Here's how the part is built. I have some questions about the finished solid (model axes, mm). Face numbers are marked on the shaded views. A direction names the side the tool comes from. Coordinates: 2 decimals unless noted, no trailing zeros. Write each loop counter-clockwise with the first axis right and the second up, starting at its lowest first coordinate (ties: lowest second). Pieces come first, ordered by that corner, then holes. Notation, with made-up numbers: (79, -29) - (123, -29) arc R22 ccw to (123, -8) - close; hole circle Ø6 at (89.25, 32.25). An arc over 180 degrees is marked (long way). Answer in a Markdown table with one row per item. Add a question column.
Item 1: Which directions (+Z, -Z, +X, -X, +Y, -Y) give clear straight access to the entire face, cutting with the end or side of a thin tool? Please do the marked faces 1 and 2.
Item 2: If I drill on probe 1 along Y at (x, z) = (2.5, 5.25); probe 2 along Y at (x, z) = (2.5, 0.5); probe 3 along X at (y, z) = (14, -0.25), over which ranges is the centre line in solid material (lowest first)? Write a range as from..to.
Item 3: Imagine slicing it at A-A (y = 2). Please give me the cut outline in (x, z), plus the area to 3 significant figures.
Item 4: We'd pull the mould along Y, two halves only. Please class the marked faces 3, 4 and 5: +Y half, -Y half, draft (parallel to the pull), parting line (faces both ways), or undercut.
Item 5: I'm going to push flat-ended pins straight in: pin 1 (2 mm diameter, centred on x = -2.5, z = 4.5, fed in from +Y); pin 2 (0.8 mm diameter, centred on x = 2, z = -3.5, fed in from -Y); pin 3 (2 mm diameter, centred on x = 3, z = 4, fed in from +Y). Where does each tip first touch, or does it pass through?
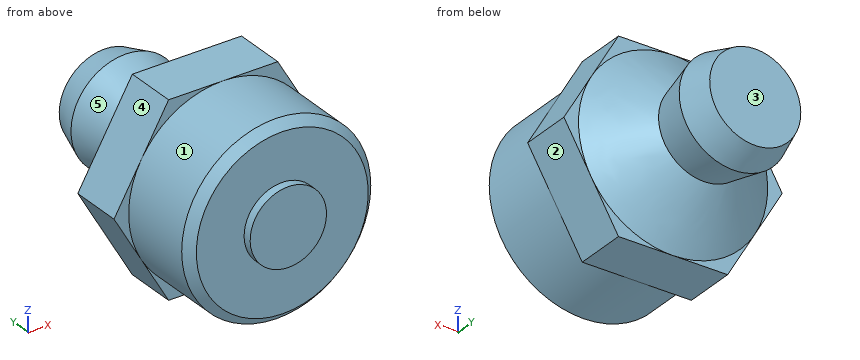
from build123d import *

# Parameters (mm, degrees)
SKETCH1_R           = 5.5
BOSS_EXTRUDE1_DEPTH = 4.89
CHAMFER1_SIZE       = 0.5
SKETCH2_R           = 2.22
BOSS_EXTRUDE2_DEPTH = 0.5
BOSS_EXTRUDE3_DEPTH = 3
SKETCH4_R           = 2.65
BOSS_EXTRUDE4_DEPTH = 2.57
SKETCH8_R           = 3.195
SKETCH5_R           = 2.65


with BuildPart() as part:
    # Sketch1 → Boss-Extrude1 (new body)
    with BuildSketch(Plane(origin=(0, 0, 0), x_dir=(1, 0, 0), z_dir=(0, 1, 0))):
        with Locations(Location((0, 0, 0), (0, 0, 270))):
            Circle(SKETCH1_R)
    extrude(amount=BOSS_EXTRUDE1_DEPTH)

    # Chamfer1
    chamfer1_edges = [part.edges().sort_by_distance(p)[0] for p in [
        (0, 0, -5.5),
    ]]
    chamfer(chamfer1_edges, length=CHAMFER1_SIZE)

    # Sketch2 → Boss-Extrude2 (add)
    with BuildSketch(Plane(origin=(0, 0, 0), x_dir=(-1, 0, 0), z_dir=(0, -1, 0))):
        with Locations(Location((0, 0, 0), (0, 0, 90))):
            Circle(SKETCH2_R)
    extrude(amount=BOSS_EXTRUDE2_DEPTH)

    # Sketch3 → Boss-Extrude3 (add)
    with BuildSketch(Plane(origin=(0, 4.89, 0), x_dir=(1, 0, 0), z_dir=(0, 1, 0))):
        Polygon((-6.350852961, 0), (-3.175426481, -5.5), (3.175426481, -5.5), (6.350852961, 0), (3.175426481, 5.5), (-3.175426481, 5.5), align=None)
    extrude(amount=BOSS_EXTRUDE3_DEPTH)

    # Sketch4 → Boss-Extrude4 (add)
    with BuildSketch(Plane(origin=(0, 7.89, 0), x_dir=(1, 0, 0), z_dir=(0, 1, 0))):
        with Locations(Location((0, 0, 0), (0, 0, 270))):
            Circle(SKETCH4_R)
    extrude(amount=BOSS_EXTRUDE4_DEPTH)

    # Loft1: read off the stored shape, not the designer's step
    # Loft1: loft between two sections, ruled curve by curve
    loft1_from = [
        Edge.make_bspline([(2.920740302, 7.89, 4.660394413), (12.241529129, 7.89, -1.181086191), (6.400048524, 7.89, -10.501875018), (-2.920740302, 7.89, -4.660394413), (-12.241529129, 7.89, 1.181086191), (-6.400048524, 7.89, 10.501875018), (2.920740302, 7.89, 4.660394413)], [0, 0, 0, 0, 0.5, 0.5, 0.5, 1, 1, 1, 1], 3, [1, 0.333333333, 0.333333333, 1, 0.333333333, 0.333333333, 1]),
    ]
    loft1_to = [
        Edge.make_bspline([(1.954409761, 10.46, 1.789631942), (5.533673644, 10.46, -2.11918758), (1.624854122, 10.46, -5.698451464), (-1.954409761, 10.46, -1.789631942), (-5.533673644, 10.46, 2.11918758), (-1.624854122, 10.46, 5.698451464), (1.954409761, 10.46, 1.789631942)], [0, 0, 0, 0, 0.5, 0.5, 0.5, 1, 1, 1, 1], 3, [1, 0.333333333, 0.333333333, 1, 0.333333333, 0.333333333, 1]),
    ]
    loft1 = Solid(Shell([*[Face.make_surface_from_curves(loft1_from[k], loft1_to[k]) for k in range(1)], Face(Wire(loft1_from)), Face(Wire(loft1_to))]))
    add(loft1)

    # Sketch8 → section 1 of loft2
    with BuildSketch(Plane(origin=(0, 12.94, 0), x_dir=(1, 0, 0), z_dir=(0, 1, 0)), mode=Mode.PRIVATE) as loft2_s1:
        Circle(SKETCH8_R)
    # loft up to a face of the part (loft2)
    loft([Face(Wire([part.edges().sort_by_distance((-0.033300005, 10.46, -2.649790767))[0]])), loft2_s1.sketch])

    # Sketch5 → section 1 of loft3
    with BuildSketch(Plane(origin=(0, 14.69, 0), x_dir=(1, 0, 0), z_dir=(0, 1, 0)), mode=Mode.PRIVATE) as loft3_s1:
        Circle(SKETCH5_R)
    # loft up to a face of the part (loft3)
    loft([Face(Wire([part.edges().sort_by_distance((-0.040148497, 12.94, -3.194747736))[0]])), loft3_s1.sketch])


solid = part.part
Here are the results:
| question | item | result |
|---|---|---|
| 1 | face 1 | -Y |
| 1 | face 2 | -Z, +X, +Y, -Y |
| 2 | probe 1 | y = 4.89..7.89 |
| 2 | probe 2 | y = 0..14.69 |
| 2 | probe 3 | x = -2.85..2.85 |
| 3 | outline | circle Ø11 at (0, 0) |
| 3 | area | 95.0 mm2 |
| 4 | face 3 | +Y half |
| 4 | face 4 | draft |
| 4 | face 5 | undercut |
| 5 | pin 1 | stops at y = 9.08 |
| 5 | pin 2 | stops at y = 0 |
| 5 | pin 3 | stops at y = 9.21 |
